Verification items for the finished model (mm, model axes). A direction names the side the tool comes from. Round coordinates to 2 decimals unless told otherwise and drop trailing zeros. Answer in a Markdown table with one row per item. Add a question column.
```python
from build123d import *

# Parameters (mm, degrees)
BOSS_EXTRUDE1_DEPTH   = 20
SKETCH1_3_R           = 10
BOSS_EXTRUDE2_DEPTH   = 10
F_1_0MM_DOWEL_HOLE1_D = 10
CRVPATTERN1_OUTLINE_R = 5
CRVPATTERN1_DEPTH     = 20
FILLET1_R             = 0.5


# Read off the part's stored shape, not the designer's step: CrvPattern1
with BuildPart() as part:
    # Sketch1 → Boss-Extrude1 (new body)
    with BuildSketch(Plane.XY):
        with BuildLine():
            Line((-44.845, -96), (44.845, -96))
            ThreePointArc((44.845, -96), (140.845, 0), (44.845, 96))
            Line((44.845, 96), (-44.845, 96))
            ThreePointArc((-44.845, 96), (-140.845, 0), (-44.845, -96))
        make_face()
        with BuildLine():
            ThreePointArc((0, -53.422733691), (114.595, 0), (0, 53.422733691))
            ThreePointArc((0, 53.422733691), (-114.595, 0), (0, -53.422733691))
        make_face(mode=Mode.SUBTRACT)
    extrude(amount=BOSS_EXTRUDE1_DEPTH)

    # Sketch1<3> → Boss-Extrude2 (add)
    with BuildSketch(Plane.XY):
        with BuildLine():
            ThreePointArc((0, 53.422733691), (-114.595, 0), (0, -53.422733691))
            ThreePointArc((0, -53.422733691), (114.595, 0), (0, 53.422733691))
        make_face()
        with Locations((44.845, 0)):
            Circle(SKETCH1_3_R, mode=Mode.SUBTRACT)
        with Locations((-44.845, 0)):
            Circle(SKETCH1_3_R, mode=Mode.SUBTRACT)
    extrude(amount=BOSS_EXTRUDE2_DEPTH)

    # Ø1.0mm Dowel Hole1 (through all)
    with Locations(Plane.XY.offset(20)):
        with Locations((127.72, 0)):
            Hole(F_1_0MM_DOWEL_HOLE1_D / 2)

    # CrvPattern1 outline → CrvPattern1 (cut)
    with BuildSketch(Plane.XY):
        with Locations((113.085024418, 47.027276047)):
            Circle(CRVPATTERN1_OUTLINE_R)
        with Locations((74.348906367, 77.445368707)):
            Circle(CRVPATTERN1_OUTLINE_R)
        with Locations((25.003535083, 82.875)):
            Circle(CRVPATTERN1_OUTLINE_R)
        with Locations((-25.003535083, 82.875)):
            Circle(CRVPATTERN1_OUTLINE_R)
        with Locations((-74.348906367, 77.445368707)):
            Circle(CRVPATTERN1_OUTLINE_R)
        with Locations((-113.085024418, 47.027276047)):
            Circle(CRVPATTERN1_OUTLINE_R)
        with Locations((-127.72, 0)):
            Circle(CRVPATTERN1_OUTLINE_R)
        with Locations((-113.085024418, -47.027276047)):
            Circle(CRVPATTERN1_OUTLINE_R)
        with Locations((-74.348906367, -77.445368707)):
            Circle(CRVPATTERN1_OUTLINE_R)
        with Locations((-25.003535083, -82.875)):
            Circle(CRVPATTERN1_OUTLINE_R)
        with Locations((25.003535083, -82.875)):
            Circle(CRVPATTERN1_OUTLINE_R)
        with Locations((74.348906367, -77.445368707)):
            Circle(CRVPATTERN1_OUTLINE_R)
        with Locations((113.085024418, -47.027276047)):
            Circle(CRVPATTERN1_OUTLINE_R)
    extrude(amount=CRVPATTERN1_DEPTH, mode=Mode.SUBTRACT)

    # Fillet1
    fillet1_edges = [part.edges().sort_by_distance(p)[0] for p in [
        (-114.595, 0, 20),
        (0, 53.422733691, 15),
        (0, -53.422733691, 15),
        (0, -96, 20),
        (140.845, 0, 20),
        (-114.595, 0, 10),
        (114.595, 0, 10),
        (0, 96, 20),
        (-140.845, 0, 20),
        (114.595, 0, 20),
    ]]
    fillet(fillet1_edges, radius=FILLET1_R)


solid = part.part
```
1) Thickness scan on L1, parallel to X at y = 49, z = 8.75; L2, parallel to X at y = 56, z = 12; L3, parallel to Y at x = 109.5, z = 14.25. Record the ranges inside material, lowest first. Write a range as [from, to].
2) Cross-section at A-A, the plane z = 2.75. Give the number of separate pieces and of enclosed holes in the cut face, and give its area (3 significant figures).
3) Draft check along Y on faces 1 (the face through (-1, -63, 20)), 2 (the face through (-1, -96, 10)), 3 (the face through (-79.344, -77.226, 9.86)), 4 (the face through (76.66, 73.01, 9.86)). Enter one of: +Y half, -Y half, draft (parallel to the pull), parting line (faces both ways), or undercut.
4) Tool access check on faces 5 (the face through (-78.317, 74.403, 9.86)), 6 (the face through (114.56, -2.21, 14.94)). Record the directions out of +Z, -Z, +X, -X, +Y, -Y that give a thin tool (end or side, any length) a straight path to the whole face; none if there is none.
5) Depth check by flat-ended pin: P1, Ø13, axis at x = 74.35, y = -77.45, coming from the +Z side; P2, Ø10, axis at y = -65, z = 16.5, coming from the -X side (3 decimals); P3, Ø23, axis at x = 44.845, y = 0, coming from the +Z side; P4, Ø1, axis at y = -43.5, z = 4, coming from the -X side. Enter the tip coordinate at first touch or a pass-through.
Results below:
| question | item | result |
|---|---|---|
| 1 | L1 | [-127.4, -117.68], [-108.49, 108.49], [117.68, 127.4] |
| 1 | L2 | [-122.82, -86.43], [-3.26, 3.26], [86.43, 122.82] |
| 1 | L3 | [-70.96, -50.51], [-43.54, -26.17], [26.17, 43.54], [50.51, 70.96] |
| 2 | separate pieces | 1 |
| 2 | enclosed holes | 16 |
| 2 | area | 44,400 mm² |
| 3 | face 1 | draft |
| 3 | face 2 | -Y half |
| 3 | face 3 | undercut |
| 3 | face 4 | undercut |
| 4 | face 5 | +Z, -Z |
| 4 | face 6 | +Z |
| 5 | P1 | z = 20 |
| 5 | P2 | x = -119.785 |
| 5 | P3 | z = 10 |
| 5 | P4 | x = -130.68 |
